CAD build for the part. Positions are in the model's coordinates, mm. Round coordinates to 2 decimals unless told otherwise and drop trailing zeros. Write each loop counter-clockwise with the first axis right and the second up, starting at its lowest first coordinate (ties: lowest second). Pieces come first, ordered by that corner, then holes. Notation, with made-up numbers: (63, 54.25) - (115, 54.25) arc R15 cw to (115, 60.25) - close; hole circle Ø5 at (-34.75, -12). An arc over 180 degrees is marked (long way). Put each result on its own line as item: value. Start each with the question number.
Item 1: Drill centre lines: line 1 (Y direction, x = 15, z = -1.1); line 2 (X direction, y = -75, z = -1.4); line 3 (Y direction, x = 77, z = -0.5). Where is each one in solid material? Low to high. Write a range as from..to.
Item 2: Cut at A-A (x = 15). Give the cut face in (y, z), and give its area (3 significant figures).
Item 3: Cut at B-B (y = -15). Give the cut face in (x, z), and give its area (3 significant figures).
Item 4: Cut at C-C (z = -0.45). Count the separate pieces of the cut face and the enclosed holes in it, and give its area (3 significant figures).
Item 5: Cut at D-D (x = 75). Give the cut face in (y, z), and give its area (3 significant figures).
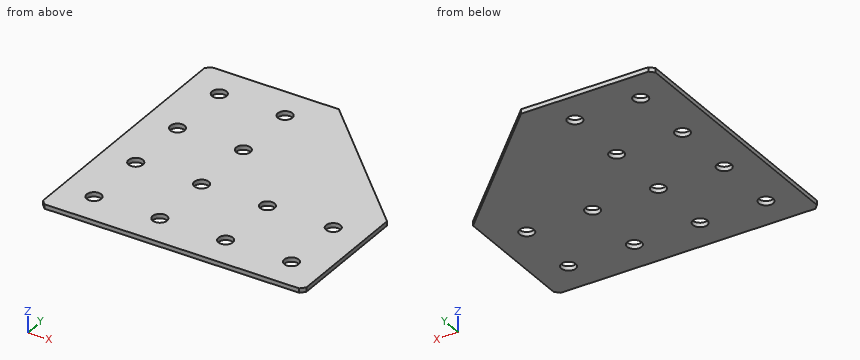
```python
from build123d import *

# Parameters (mm, degrees)
EXTRUDE_1_DEPTH   = 2
HOLE_WIZARD_M61_D = 6.6
CHAMFER_1_SIZE    = 2


with BuildPart() as part:
    # Эскиз1 → Бобышка-Вытянуть1 (new body)
    with BuildSketch(Plane(origin=(0, 0, 0), x_dir=(1, 0, 0), z_dir=(0, 0, -1))):
        Polygon((0, 0), (0, 120), (120, 120), (120, 60), (60, 0), align=None)
    extrude(amount=EXTRUDE_1_DEPTH)

    # Отверстие с зазором M61 (through all)
    with Locations(Plane(origin=(0, 0, -2), x_dir=(1, 0, 0), z_dir=(0, 0, -1))):
        with Locations((15, 105), (15, 75), (15, 45), (15, 15), (45, 105), (45, 75), (45, 45), (45, 15), (75, 105), (75, 75), (105, 105), (105, 75)):
            Hole(HOLE_WIZARD_M61_D / 2)

    # Фаска1
    chamfer_1_edges = [part.edges().sort_by_distance(p)[0] for p in [
        (0, 0, -1),
        (0, -120, -1),
        (120, -120, -1),
    ]]
    chamfer(chamfer_1_edges, length=CHAMFER_1_SIZE)


solid = part.part
```
Output values:
1. line 1: -120..-108.3, -101.7..-78.3, -71.7..-48.3, -41.7..-18.3, -11.7..0
1. line 2: 0..11.7, 18.3..41.7, 48.3..71.7, 78.3..101.7, 108.3..120
1. line 3: -120..-107.62, -102.38..-77.62, -72.38..-17
2. outline: (-120, -2) - (-108.3, -2) - (-108.3, 0) - (-120, 0) - close; (-101.7, -2) - (-78.3, -2) - (-78.3, 0) - (-101.7, 0) - close; (-71.7, -2) - (-48.3, -2) - (-48.3, 0) - (-71.7, 0) - close; (-41.7, -2) - (-18.3, -2) - (-18.3, 0) - (-41.7, 0) - close; (-11.7, -2) - (0, -2) - (0, 0) - (-11.7, 0) - close
2. area: 187 mm2
3. outline: (0, -2) - (11.7, -2) - (11.7, 0) - (0, 0) - close; (18.3, -2) - (41.7, -2) - (41.7, 0) - (18.3, 0) - close; (48.3, -2) - (75, -2) - (75, 0) - (48.3, 0) - close
3. area: 124 mm2
4. separate pieces: 1
4. enclosed holes: 12
4. area: 12,200 mm2
5. outline: (-120, -2) - (-108.3, -2) - (-108.3, 0) - (-120, 0) - close; (-101.7, -2) - (-78.3, -2) - (-78.3, 0) - (-101.7, 0) - close; (-71.7, -2) - (-15, -2) - (-15, 0) - (-71.7, 0) - close
5. area: 184 mm2
